Geometry check sheet. Reference: the model listing, model coordinates, mm. Round coordinates to 2 decimals unless told otherwise and drop trailing zeros. Order: outer loops, then holes, each group sorted by start corner. A loop starts at its lowest first (then second) coordinate and runs counter-clockwise, first axis right, second up. Notation, with made-up numbers: (14.25, -5) - (47.25, -5) arc R13 ccw to (47.25, 14) - close; hole circle Ø11 at (88.5, 83). An arc over 180 degrees is marked (long way). Return JSON: item names as keys, results as strings. Group by question number.
Q1. Sectioned sample at A-A, the plane z = 113.5. Record the cut outline in (x, y), then the cut area to 3 significant figures.
Q2. Sectioned sample at B-B, the plane y = 4. Record the cut outline in (x, z), then the cut area to 3 significant figures.
Q3. Material ranges on line 1 along Y through (x, z) = (0, 539); line 2 along X through (y, z) = (-0.5, 87); line 3 along Y through (x, z) = (-1.75, 272), recorded low to high.
Q4. Gauge pin test, flat ends, axial feed: pin 1 Ø3 at (y, z) = (-3.5, 150.5) entering from -X; pin 2 Ø1.5 at (y, z) = (-3, 459.5) entering from +X; pin 3 Ø1.5 at (y, z) = (2, 94) entering from +X. Record the tip position at first contact, or that the pin passes through.
```python
from build123d import *

# Parameters (mm, degrees)
SKETCH1_R                  = 6.4
BOSS_EXTRUDE1_DEPTH        = 548.24
F_10_24_TAPPED_HOLE1_D     = 3.7973
F_10_24_TAPPED_HOLE1_DEPTH = 12.83
F_10_24_TAPPED_HOLE1_TIP   = 1.140824014
F_10_24_TAPPED_HOLE2_D     = 3.7973
F_10_24_TAPPED_HOLE2_DEPTH = 12.83
F_10_24_TAPPED_HOLE2_TIP   = 1.140824014


with BuildPart() as part:
    # Sketch1 → Boss-Extrude1 (new body)
    with BuildSketch(Plane.XY):
        Circle(SKETCH1_R)
    extrude(amount=BOSS_EXTRUDE1_DEPTH)

    # #10-24 Tapped Hole1
    with Locations(Plane(origin=(0, 0, 0), x_dir=(-1, 0, 0), z_dir=(0, 0, -1))):
        with Locations((0, 0)):
            Hole(F_10_24_TAPPED_HOLE1_D / 2, depth=F_10_24_TAPPED_HOLE1_DEPTH)
            with Locations((0, 0, -(F_10_24_TAPPED_HOLE1_DEPTH + F_10_24_TAPPED_HOLE1_TIP / 2))):  # 118° drill point
                Cone(0, F_10_24_TAPPED_HOLE1_D / 2, F_10_24_TAPPED_HOLE1_TIP, mode=Mode.SUBTRACT)

    # #10-24 Tapped Hole2
    with Locations(Plane.XY.offset(548.24)):
        with Locations((0, 0)):
            Hole(F_10_24_TAPPED_HOLE2_D / 2, depth=F_10_24_TAPPED_HOLE2_DEPTH)
            with Locations((0, 0, -(F_10_24_TAPPED_HOLE2_DEPTH + F_10_24_TAPPED_HOLE2_TIP / 2))):  # 118° drill point
                Cone(0, F_10_24_TAPPED_HOLE2_D / 2, F_10_24_TAPPED_HOLE2_TIP, mode=Mode.SUBTRACT)


solid = part.part
```
Reply:
{
 "1": {"outline": "circle Ø12.8 at (0, 0)", "area": "129 mm^2"},
 "2": {"outline": "(-5, 0) - (5, 0) - (5, 548.24) - (-5, 548.24) - close", "area": "5,480 mm^2"},
 "3": {"line 1": "-6.4 to -1.9, 1.9 to 6.4", "line 2": "-6.38 to 6.38", "line 3": "-6.16 to 6.16"},
 "4": {"pin 1": "x = -6.08", "pin 2": "x = 5.99", "pin 3": "x = 6.28"}
}
